Check sheet for the modelled part. Datum: model origin and axes. Units: mm. Face numbers are marked on the shaded views. A direction names the side the tool comes from. Give positions to 0.01 mm unless a question says otherwise; leave off trailing zeros. Write each loop counter-clockwise with the first axis right and the second up, starting at its lowest first coordinate (ties: lowest second). Pieces come first, ordered by that corner, then holes. Notation, with made-up numbers: M 71,52 L 129,52 A8 ccw 129,56 Z; hole C -8.5,16 d1. An arc over 180 degrees is marked long. Use CSV: the item, a comma, the result in double quotes. Start each with the question number.
1. Access from +Z, -Z, +X, -X, +Y, -Y to the whole of each face (thin tool, end or side, straight path). Record for the marked faces 1, 2, 3 and 4.
2. Scan lines: line 1 (X direction, y = -19.5, z = 68); line 2 (Z direction, x = 4.5, y = 3); line 3 (Y direction, x = -16, z = 43). Record each from-to range of solid material in increasing order.
3. Depth check by flat-ended pin: P1, Ø4, axis at x = -11.5, z = 16, coming from the -Y side; P2, Ø3, axis at x = -11, y = 11.5, coming from the +Z side; P3, Ø3.5, axis at x = -12.5, y = -20, coming from the -Z side; P4, Ø5.5, axis at x = -16, z = 5.5, coming from the -Y side. Enter the tip coordinate at first touch or a pass-through.
4. Cross-section at D-D, the plane x = 0. Enter the section's corners in (y, z).
5. Cross-section at C-C, the plane y = -21. Enter the section's corners in (x, z).
6. Cross-section at B-B, the plane z = 56. Enter the section's corners in (x, y), and give its area (3 significant figures).
7. Cross-section at A-A, the plane x = -13.5. Enter the section's corners in (y, z).
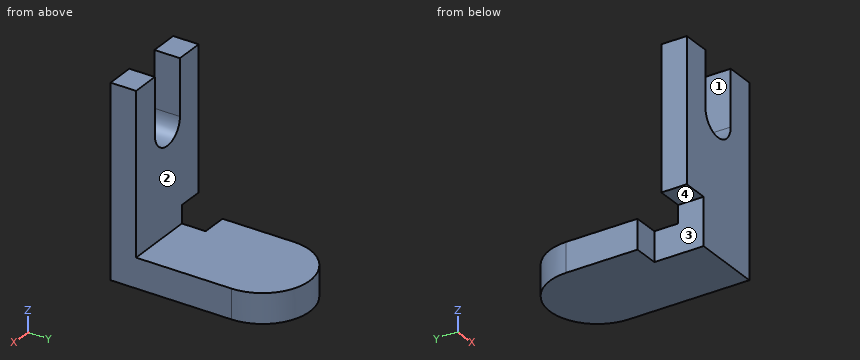
from build123d import *

# Parameters (mm, degrees)
F1_DEPTH = 12.7
F2_W     = 40.6866073608
F2_H     = 10.9301833436
F3_DEPTH = 68.58
F5_DEPTH = 25.4
F7_DEPTH = 10.922


with BuildPart() as f1:
    # F0 (on Top) → F1 (new body)
    with BuildSketch(Plane.XY):
        with BuildLine():
            Line((-20.3433036804, -25.90101026), (20.3433036804, -25.90101026))
            Line((20.3433036804, -25.90101026), (20.3433036804, 25.90101026))
            ThreePointArc((20.3433036804, 25.90101026), (0, 46.2443139404), (-20.3433036804, 25.90101026))
            Line((-20.3433036804, 25.90101026), (-20.3433036804, -25.90101026))
        make_face()
    extrude(amount=F1_DEPTH)

    # F2 (on face) → F3 (join)
    with BuildSketch(Plane.XY.offset(12.7)):
        with Locations((0, -20.4359185882)):
            Rectangle(F2_W, F2_H)
    extrude(amount=F3_DEPTH)

    # F4 (on face) → F5 (cut)
    with BuildSketch(Plane(origin=(0, -14.9708269164, 0), x_dir=(-1, 0, 0), z_dir=(0, 1, 0))):
        with BuildLine():
            Line((8.1715718843, 81.28), (-8.1715718843, 81.28))
            Line((-8.1715718843, 81.28), (-8.1715718843, 57.2796314955))
            ThreePointArc((-8.1715718843, 57.2796314955), (0, 49.1080596112), (8.1715718843, 57.2796314955))
            Line((8.1715718843, 57.2796314955), (8.1715718843, 81.28))
        make_face()
    extrude(amount=-F5_DEPTH, mode=Mode.SUBTRACT)

    # F6 (on face) → F7 (cut)
    with BuildSketch(Plane(origin=(-20.3433036804, 0, 0), x_dir=(0, -1, 0), z_dir=(-1, 0, 0))):
        Polygon((4.7405310906, 0), (25.90101026, 0), (25.90101026, 20.310420543), (14.9708269164, 20.310420543), (14.9708269164, 12.7), (4.7405310906, 12.7), align=None)
    extrude(amount=-F7_DEPTH, mode=Mode.SUBTRACT)


solid = f1.part
Worked answers:
1,face 1,"+Z, +Y, -Y"
1,face 2,"+Z, +X, -X, +Y"
1,face 3,"-Z, -X, -Y"
1,face 4,"-Z, -X, +Y, -Y"
2,line 1,"x = -20.34 to -8.17, 8.17 to 20.34"
2,line 2,"z = 0 to 12.7"
2,line 3,"y = -25.9 to -14.97"
3,P1,"passes through"
3,P2,"stops at z = 12.7"
3,P3,"stops at z = 20.31"
3,P4,"stops at y = -4.74"
4,outline,"M -25.9,0 L 46.24,0 L 46.24,12.7 L -14.97,12.7 L -14.97,49.11 L -25.9,49.11 Z"
5,outline,"M -20.34,20.31 L -9.42,20.31 L -9.42,0 L 20.34,0 L 20.34,81.28 L 8.17,81.28 L 8.17,57.28 A8.17 cw -8.17,57.28 L -8.17,81.28 L -20.34,81.28 Z"
6,outline,"M -20.34,-25.9 L -8.07,-25.9 L -8.07,-14.97 L -20.34,-14.97 Z; M 8.07,-25.9 L 20.34,-25.9 L 20.34,-14.97 L 8.07,-14.97 Z"
6,area,"268 mm^2"
7,outline,"M -25.9,20.31 L -14.97,20.31 L -14.97,81.28 L -25.9,81.28 Z; M -4.74,0 L 41.12,0 L 41.12,12.7 L -4.74,12.7 Z"
